The figure shows three views and two pictorial views of one solid part (mm, origin at its lowest corner). Answer the questions. Coordinates: 2 decimals unless noted, no trailing zeros. Write each loop counter-clockwise with the first axis right and the second up, starting at its lowest first coordinate (ties: lowest second). Pieces come first, ordered by that corner, then holes. Notation, with made-up numbers: M 79,-38 L 102,-38 A25 cw 102,-21 Z; hole C 23.25,-11.75 d10. An arc over 180 degrees is marked long. Write item = value, one per line.
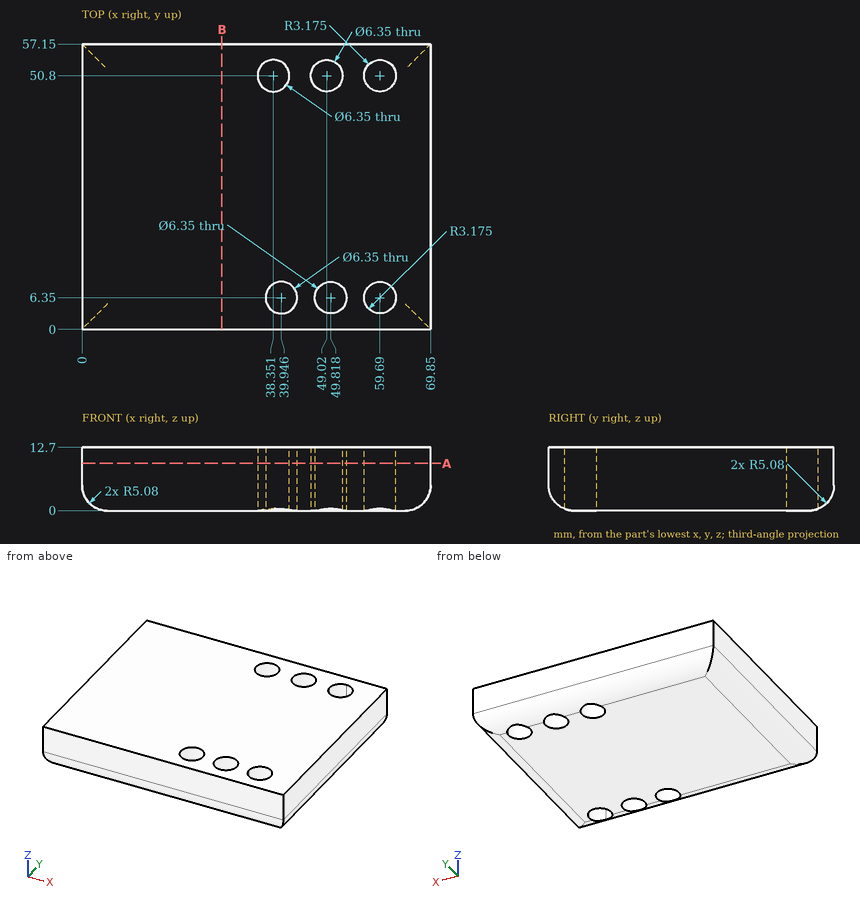
Item 1: Find section A-A (z = 9.5). State how many separate pieces and enclosed holes the cut face has, and give its area (3 significant figures).
Worked answers:
separate_pieces = 1
enclosed_holes = 6
area = 3,800 mm²
Item 2: Consider line 1 along X through (y, z) = (53, 7); line 2 along Z through (x, y) = (65, 40.5) (1 decimal); line 3 along Y through (x, z) = (64, 2). Determine where each line is inside the solid, lowest interval first. Write a range as from..to.
Worked answers:
line_1 = 0..36.06, 40.64..46.73, 51.31..57.4, 61.98..69.85
line_2 = 0..12.7
line_3 = 1.04..56.11
Item 3: Find section B-B (x = 28). Determine the outline of the cut face in (y, z), and give its area (3 significant figures).
Worked answers:
outline = M 0,5.08 A5.08 ccw 5.08,0 L 52.07,0 A5.08 ccw 57.15,5.08 L 57.15,12.7 L 0,12.7 Z
area = 715 mm²
